Drawing for the job (mm, zero at the part's lowest x, y, z). Give positions to 0.01 mm unless a question says otherwise; leave off trailing zeros. Loops run counter-clockwise (first coordinate to the right, second up) from the corner with the lowest first, then second, coordinate; pieces in that order, holes last.
1) Band-saw the part on B-B on x = 38.1. List the corners of the cut face in (y, z) (1 decimal).
2) Band-saw the part on A-A on x = 69.85. List the corners of the cut face in (y, z) (1 decimal).
3) Band-saw the part on C-C on z = 2.3. State how many separate pieces and enclosed holes the cut face has, then the cut area to 3 significant figures.
4) Flat gauge pin, fed straight in: P1, Ø4.5, axis at x = 6.35, y = 6.35, coming from the +Z side. Where does the tip first touch, or does it go through?
5) Wall check: line 1 (Y direction, x = 69.85, z = 1.4); line 2 (Y direction, x = 38.1, z = 4.5); line 3 (Y direction, x = 69, z = 5.25). Give the ranges that are in metal, low to high.
6) Band-saw the part on D-D on y = 25.4. List the corners of the cut face in (x, z) (1 decimal), then the cut area to 3 significant figures.
7) Two-plate mould, pull along X, no slides. Class the marked faces 1 and 2: +X half, -X half, draft (parallel to the pull), parting line (faces both ways), or undercut.
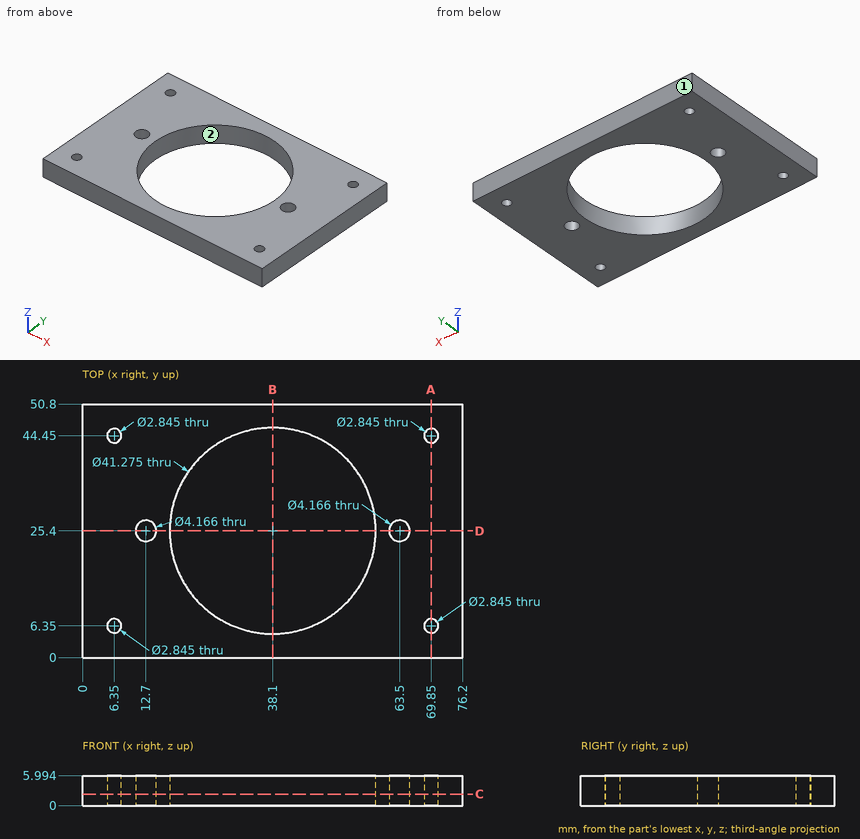
Findings below:
1. outline: (0, 0) - (4.8, 0) - (4.8, 6) - (0, 6) - close; (46, 0) - (50.8, 0) - (50.8, 6) - (46, 6) - close
2. outline: (0, 0) - (4.9, 0) - (4.9, 6) - (0, 6) - close; (7.8, 0) - (43, 0) - (43, 6) - (7.8, 6) - close; (45.9, 0) - (50.8, 0) - (50.8, 6) - (45.9, 6) - close
3. separate pieces: 1
3. enclosed holes: 7
3. area: 2,480 mm2
4. P1: stops at z = 5.99
5. line 1: y = 0 to 4.93, 7.77 to 43.03, 45.87 to 50.8
5. line 2: y = 0 to 4.76, 46.04 to 50.8
5. line 3: y = 0 to 5.21, 7.49 to 43.31, 45.59 to 50.8
6. outline: (0, 0) - (10.6, 0) - (10.6, 6) - (0, 6) - close; (14.8, 0) - (17.5, 0) - (17.5, 6) - (14.8, 6) - close; (58.7, 0) - (61.4, 0) - (61.4, 6) - (58.7, 6) - close; (65.6, 0) - (76.2, 0) - (76.2, 6) - (65.6, 6) - close
6. area: 159 mm2
7. face 1: draft
7. face 2: undercut
